Work out the finished part from the listing and answer in its coordinate system (mm). Give positions to 0.01 mm unless a question says otherwise; leave off trailing zeros. Order: outer loops, then holes, each group sorted by start corner. A loop starts at its lowest first (then second) coordinate and runs counter-clockwise, first axis right, second up.
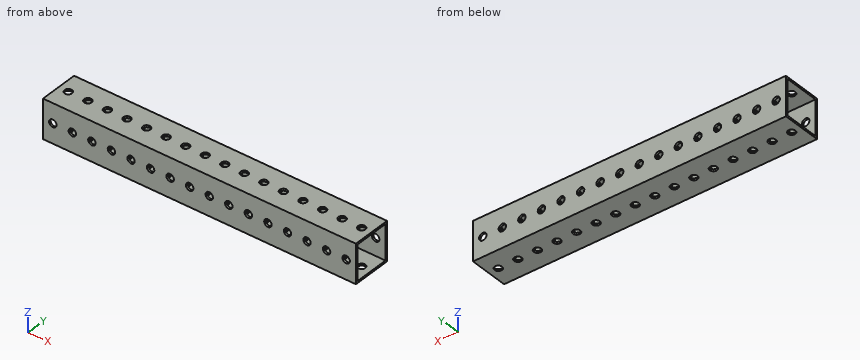
```python
from build123d import *

# Parameters (mm, degrees)
SKETCH1_W           = 203.2
SKETCH1_H           = 25.4
BOSS_EXTRUDE1_DEPTH = 25.4
SKETCH2_W           = 22.86
SKETCH2_H           = 22.86
CUT_EXTRUDE1_DEPTH  = 207.350575478
SKETCH3_R           = 2.413
CUT_EXTRUDE2_DEPTH  = 207.350575478
SKETCH4_R           = 2.413
CUT_EXTRUDE3_DEPTH  = 207.350575478


with BuildPart() as part:
    # Sketch1 → Boss-Extrude1 (new body)
    with BuildSketch(Plane(origin=(0, 0, 0), x_dir=(1, 0, 0), z_dir=(0, 1, 0))):
        with Locations((101.6, 12.7)):
            Rectangle(SKETCH1_W, SKETCH1_H)
    extrude(amount=BOSS_EXTRUDE1_DEPTH)

    # Sketch2 → Cut-Extrude1 (cut, through all)
    with BuildSketch(Plane.ZY):
        with Locations((-12.7, 12.7)):
            Rectangle(SKETCH2_W, SKETCH2_H)
    extrude(amount=-CUT_EXTRUDE1_DEPTH, mode=Mode.SUBTRACT)

    # Sketch3 → Cut-Extrude2 (cut, through all)
    with BuildSketch(Plane(origin=(0, 25.4, 0), x_dir=(1, 0, 0), z_dir=(0, 1, 0))):
        with Locations(Location((6.35, 12.7, 0), (0, 0, 270))):
            Circle(SKETCH3_R)
        with Locations(Location((19.05, 12.7, 0), (0, 0, 270))):
            Circle(SKETCH3_R)
        with Locations(Location((31.75, 12.7, 0), (0, 0, 270))):
            Circle(SKETCH3_R)
        with Locations(Location((44.45, 12.7, 0), (0, 0, 270))):
            Circle(SKETCH3_R)
        with Locations(Location((57.15, 12.7, 0), (0, 0, 270))):
            Circle(SKETCH3_R)
        with Locations(Location((69.85, 12.7, 0), (0, 0, 270))):
            Circle(SKETCH3_R)
        with Locations(Location((82.55, 12.7, 0), (0, 0, 270))):
            Circle(SKETCH3_R)
        with Locations(Location((95.25, 12.7, 0), (0, 0, 270))):
            Circle(SKETCH3_R)
        with Locations(Location((107.95, 12.7, 0), (0, 0, 270))):
            Circle(SKETCH3_R)
        with Locations(Location((120.65, 12.7, 0), (0, 0, 270))):
            Circle(SKETCH3_R)
        with Locations(Location((133.35, 12.7, 0), (0, 0, 270))):
            Circle(SKETCH3_R)
        with Locations(Location((146.05, 12.7, 0), (0, 0, 270))):
            Circle(SKETCH3_R)
        with Locations(Location((158.75, 12.7, 0), (0, 0, 270))):
            Circle(SKETCH3_R)
        with Locations(Location((171.45, 12.7, 0), (0, 0, 270))):
            Circle(SKETCH3_R)
        with Locations(Location((184.15, 12.7, 0), (0, 0, 270))):
            Circle(SKETCH3_R)
        with Locations(Location((196.85, 12.7, 0), (0, 0, 270))):
            Circle(SKETCH3_R)
    extrude(amount=-CUT_EXTRUDE2_DEPTH, mode=Mode.SUBTRACT)

    # Sketch4 → Cut-Extrude3 (cut, through all)
    with BuildSketch(Plane(origin=(0, 0, -25.4), x_dir=(-1, 0, 0), z_dir=(0, 0, -1))):
        with Locations((-6.35, 12.7)):
            Circle(SKETCH4_R)
        with Locations((-19.05, 12.7)):
            Circle(SKETCH4_R)
        with Locations((-31.75, 12.7)):
            Circle(SKETCH4_R)
        with Locations((-44.45, 12.7)):
            Circle(SKETCH4_R)
        with Locations((-57.15, 12.7)):
            Circle(SKETCH4_R)
        with Locations((-69.85, 12.7)):
            Circle(SKETCH4_R)
        with Locations((-82.55, 12.7)):
            Circle(SKETCH4_R)
        with Locations((-95.25, 12.7)):
            Circle(SKETCH4_R)
        with Locations((-107.95, 12.7)):
            Circle(SKETCH4_R)
        with Locations((-120.65, 12.7)):
            Circle(SKETCH4_R)
        with Locations((-133.35, 12.7)):
            Circle(SKETCH4_R)
        with Locations((-146.05, 12.7)):
            Circle(SKETCH4_R)
        with Locations((-158.75, 12.7)):
            Circle(SKETCH4_R)
        with Locations((-171.45, 12.7)):
            Circle(SKETCH4_R)
        with Locations((-184.15, 12.7)):
            Circle(SKETCH4_R)
        with Locations((-196.85, 12.7)):
            Circle(SKETCH4_R)
    extrude(amount=-CUT_EXTRUDE3_DEPTH, mode=Mode.SUBTRACT)


solid = part.part
```
1. Given P1, Ø10, axis at x = 81.5, y = 11.5, coming from the -Z side, flat-ended and moving along its own axis, determine where the tip first touches the part or whether it passes through.
Findings below:
P1: stops at z = -25.4
2. The part is cut by section A-A (x = 95.25). Write down the section's boundary in (y, z).
Findings below:
outline: (0, -25.4) - (10.29, -25.4) - (10.29, -24.13) - (1.27, -24.13) - (1.27, -15.11) - (0, -15.11) - close; (0, -10.29) - (1.27, -10.29) - (1.27, -1.27) - (10.29, -1.27) - (10.29, 0) - (0, 0) - close; (15.11, -25.4) - (25.4, -25.4) - (25.4, -15.11) - (24.13, -15.11) - (24.13, -24.13) - (15.11, -24.13) - close; (15.11, -1.27) - (24.13, -1.27) - (24.13, -10.29) - (25.4, -10.29) - (25.4, 0) - (15.11, 0) - close
3. The part is cut by section C-C (z = -5.5). Write down the section's boundary in (x, y), then the cut area to 3 significant figures.
Findings below:
outline: (0, 0) - (203.2, 0) - (203.2, 1.27) - (0, 1.27) - close; (0, 24.13) - (203.2, 24.13) - (203.2, 25.4) - (0, 25.4) - close
area: 516 mm2
4. The part is cut by section B-B (y = 5.5). Write down the section's boundary in (x, z).
Findings below:
outline: (0, -25.4) - (203.2, -25.4) - (203.2, -24.13) - (0, -24.13) - close; (0, -1.27) - (203.2, -1.27) - (203.2, 0) - (0, 0) - close
5. The part is cut by section D-D (x = 152.5). Write down the section's boundary in (y, z).
Findings below:
outline: (0, -25.4) - (25.4, -25.4) - (25.4, 0) - (0, 0) - close; hole (1.27, -24.13) - (24.13, -24.13) - (24.13, -1.27) - (1.27, -1.27) - close
6. Straight lines are drawn through the part: probe 1 along Z at (x, y) = (164.5, 9.5); probe 2 along Y at (x, z) = (23.5, -20.75); probe 3 along Y at (x, z) = (95.25, -0.8). For each, find the intervals that lie inside material, in ascending order.
Findings below:
probe 1: z = -25.4 to -24.13, -1.27 to 0
probe 2: y = 0 to 1.27, 24.13 to 25.4
probe 3: y = 0 to 10.29, 15.11 to 25.4
